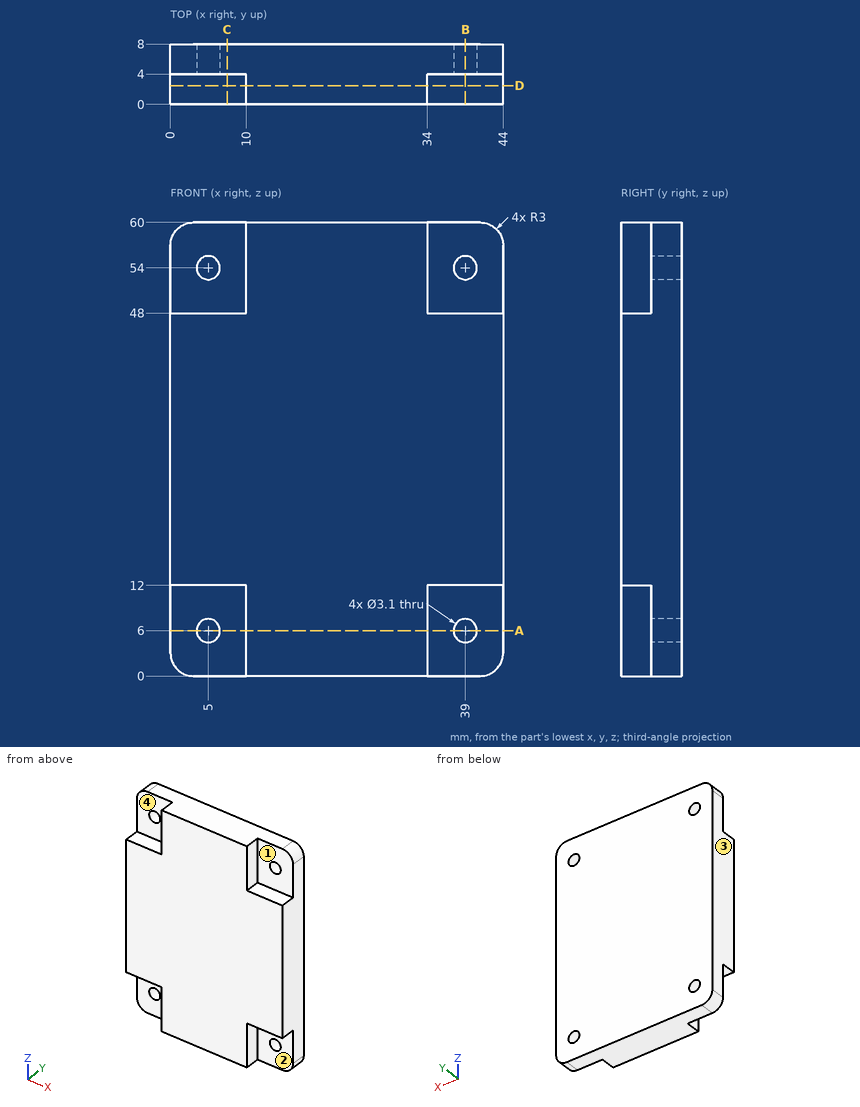
Input: dimensioned drawing with shaded views. Units: mm. Origin: part minimum x, y, z. A direction names the side the tool comes from. Give positions to 0.01 mm unless a question says otherwise; leave off trailing zeros. Loops run counter-clockwise (first coordinate to the right, second up) from the corner with the lowest first, then second, coordinate; pieces in that order, holes last. Notation, with made-up numbers: M -25,86 L -3,86 A19 ccw -3,106 Z; hole C 18,80 d4. An arc over 180 degrees is marked long. Put each result on its own line as item: value. Start each with the question number.
1) Cut plane D-D (y = 2.5). Output: boundary loops of the cut face in (x, z).
2) Ray query, line 1 along X through (y, z) = (5.1, 6); line 2 along Z through (x, y) = (5, 5.15); line 3 along X through (y, z) = (3.25, 10.5). Return the intervals inside material, ascending.
3) Cut plane A-A (z = 6). Output: boundary loops of the cut face in (x, y).
4) Cut plane C-C (x = 7.5). Output: boundary loops of the cut face in (y, z).
5) Cut plane B-B (x = 39). Output: boundary loops of the cut face in (y, z), then the cut area to 3 significant figures.
6) Access query for the marked faces 1, 2, 3 and 4. Directions: +Z, -Z, +X, -X, +Y, -Y. A direction counts if a zero-diameter tool reaches every point of the face in a straight line with its end or side. Return the directions, or none.
7) Contact query for flat-ended pins moving along their axis: pin 1 (3 mm diameter, centred on x = 41.5, y = 1, fed in from -Z); pin 2 (2 mm diameter, centred on x = 7, y = 2.5, fed in from +Z); pin 3 (8 mm diameter, centred on x = 3, z = 7, fed in from -Y). Output: stop coordinate, or through.
Verdict:
1. outline: M 0,12 L 10,12 L 10,0 L 34,0 L 34,12 L 44,12 L 44,48 L 34,48 L 34,60 L 10,60 L 10,48 L 0,48 Z
2. line 1: 0 to 3.45, 6.55 to 37.45, 40.55 to 44
2. line 2: 0 to 4.45, 7.55 to 52.45, 55.55 to 60
2. line 3: 10 to 34
3. outline: M 0,4 L 3.45,4 L 3.45,8 L 0,8 Z; M 6.55,4 L 10,4 L 10,0 L 34,0 L 34,4 L 37.45,4 L 37.45,8 L 6.55,8 Z; M 40.55,4 L 44,4 L 44,8 L 40.55,8 Z
4. outline: M 0,12 L 4,12 L 4,0 L 8,0 L 8,60 L 4,60 L 4,48 L 0,48 Z
5. outline: M 0,12 L 4,12 L 4,7.55 L 8,7.55 L 8,52.45 L 4,52.45 L 4,48 L 0,48 Z; M 4,0 L 8,0 L 8,4.45 L 4,4.45 Z; M 4,55.55 L 8,55.55 L 8,60 L 4,60 Z
5. area: 359 mm2
6. face 1: +Z, +X, -Y
6. face 2: -Z, +X, -Y
6. face 3: +Z, -Z, -X, +Y, -Y
6. face 4: +Z, -X, -Y
7. pin 1: z = 12
7. pin 2: z = 48
7. pin 3: y = 4
